```python
from build123d import *

# Parameters (mm, degrees)
BOSS_EXTRUDE1_DEPTH = 20
FILLET1_R           = 1
FILLET2_R           = 0.5
BOSS_EXTRUDE2_DEPTH = 20


with BuildPart() as part:
    # Sketch1 → Boss-Extrude1 (new body)
    with BuildSketch(Plane(origin=(0, 0, 0), x_dir=(1, 0, 0), z_dir=(0, 1, 0))):
        Polygon((-2.4, 4.581818182), (2.4, 4.581818182), (7, 0.381818182), (2.4, 0.381818182), (2.4, -1.618181818), (10, -1.618181818), (10, -4.618181818), (-10, -4.618181818), (-10, -1.618181818), (-2.4, -1.618181818), (-2.4, 0.381818182), (-7, 0.381818182), align=None)
    extrude(amount=BOSS_EXTRUDE1_DEPTH)

    # Fillet1
    fillet1_edges = [part.edges().sort_by_distance(p)[0] for p in [
        (7, 10, -0.381818182),
        (-7, 10, -0.381818182),
        (-2.4, 10, -4.581818182),
        (2.4, 10, -4.581818182),
    ]]
    fillet(fillet1_edges, radius=FILLET1_R)

    # Fillet2
    fillet2_edges = [part.edges().sort_by_distance(p)[0] for p in [
        (2.4, 10, -0.381818182),
        (2.4, 10, 1.618181818),
        (-2.4, 10, 1.618181818),
        (-2.4, 10, -0.381818182),
    ]]
    fillet(fillet2_edges, radius=FILLET2_R)

    # Sketch2 → Boss-Extrude2 (add)
    with BuildSketch(Plane(origin=(0, 20, 0), x_dir=(1, 0, 0), z_dir=(0, 1, 0))):
        Polygon((-7, -4.618181818), (-10, -4.618181818), (-10, -24.618181818), (10, -24.618181818), (10, -4.618181818), (7, -4.618181818), (7, -21.618181818), (-7, -21.618181818), align=None)
    extrude(amount=-BOSS_EXTRUDE2_DEPTH)


solid = part.part
```
Check sheet for the modelled part. Datum: model origin and axes. Units: mm. A direction names the side the tool comes from. Round coordinates to 2 decimals unless told otherwise and drop trailing zeros. Order: outer loops, then holes, each group sorted by start corner. A loop starts at its lowest first (then second) coordinate and runs counter-clockwise, first axis right, second up. Notation, with made-up numbers: (-14, 31.25) - (40, 31.25) arc R28 cw to (40, 60.25) - close; hole circle Ø8 at (-19.75, 56.25). An arc over 180 degrees is marked (long way). Answer as CSV lines item,"result". Start each with the question number.
1) Scan lines: probe 1 along Z at (x, y) = (-6.75, 11.5); probe 2 along X at (y, z) = (3, 21.25); probe 3 along Z at (x, y) = (2, 18.75). Record each from-to range of solid material in increasing order.
2) Draft check along X on faces 1 (the face through (-7, 10, 13)), 2 (the face through (-2.4, 9.9, 0.6)), 3 (the face through (3.87, 9.86, -3.24)). Enter one of: +X half, -X half, draft (parallel to the pull), parting line (faces both ways), or undercut.
3) Section check A-A (x = 6.25). Record the cut outline in (y, z), then the cut area to 3 significant figures.
4) Section check B-B (y = 17.25). Record the cut outline in (x, z), then the cut area to 3 significant figures.
5) Section check D-D (x = 8.5). Record the cut outline in (y, z), then the cut area to 3 significant figures.
6) Section check C-C (z = 20). Record the cut outline in (x, y).
7) Tool access check on faces 4 (the face through (-4, 10, -0.382)), 5 (the face through (10, 10, 13)), 6 (the face through (2.4, 9.9, 0.6)), 7 (the face through (0, 0, 3)), 8 (the face through (7, 10, 13)). Record the directions out of +Z, -Z, +X, -X, +Y, -Y that give a thin tool (end or side, any length) a straight path to the whole face; none if there is none.
8) Depth check by flat-ended pin: pin 1 (1 mm diameter, centred on x = 4, y = 3, fed in from -Z); pin 2 (0.8 mm diameter, centred on y = 5.5, z = 0.5, fed in from +X); pin 3 (2 mm diameter, centred on x = -7.5, y = 9, fed in from -Z). Enter the tip coordinate at first touch or a pass-through.
Determined:
1,probe 1,"1.62 to 4.62, 21.62 to 24.62"
1,probe 2,"-10 to -7, 7 to 10"
1,probe 3,"-4.58 to 4.62, 21.62 to 24.62"
2,face 1,"undercut"
2,face 2,"-X half"
2,face 3,"+X half"
3,outline,"(0, 1.62) - (20, 1.62) - (20, 4.62) - (0, 4.62) - close; (0, 21.62) - (20, 21.62) - (20, 24.62) - (0, 24.62) - close"
3,area,"120 mm^2"
4,outline,"(-10, 1.62) - (-2.9, 1.62) arc R0.5 cw to (-2.4, 1.12) - (-2.4, 0.12) arc R0.5 cw to (-2.9, -0.38) - (-4.42, -0.38) arc R1 ccw to (-5.1, -2.12) - (-2.69, -4.32) arc R1 ccw to (-2.01, -4.58) - (2.01, -4.58) arc R1 ccw to (2.69, -4.32) - (5.1, -2.12) arc R1 ccw to (4.42, -0.38) - (2.9, -0.38) arc R0.5 cw to (2.4, 0.12) - (2.4, 1.12) arc R0.5 cw to (2.9, 1.62) - (10, 1.62) - (10, 24.62) - (-10, 24.62) - close; hole (-7, 4.62) - (7, 4.62) - (7, 21.62) - (-7, 21.62) - close"
4,area,"269 mm^2"
5,outline,"(0, 1.62) - (20, 1.62) - (20, 24.62) - (0, 24.62) - close"
5,area,"460 mm^2"
6,outline,"(-10, 0) - (-7, 0) - (-7, 20) - (-10, 20) - close; (7, 0) - (10, 0) - (10, 20) - (7, 20) - close"
7,face 4,"-X, +Y, -Y"
7,face 5,"+Z, -Z, +X, +Y, -Y"
7,face 6,"+X, +Y, -Y"
7,face 7,"+Z, -Z, +X, -X, -Y"
7,face 8,"+Y, -Y"
8,pin 1,"z = -3.58"
8,pin 2,"x = 2.4"
8,pin 3,"z = 1.62"
